from build123d import *

# Parameters (mm, degrees)
SKETCH1_W           = 40
SKETCH1_H           = 40
BOSS_EXTRUDE1_DEPTH = 10
SKETCH2_R           = 1
CUT_EXTRUDE1_DEPTH  = 11
SKETCH3_R           = 19
CUT_EXTRUDE2_DEPTH  = 11


with BuildPart() as part:
    # Sketch1 → Boss-Extrude1 (new body)
    with BuildSketch(Plane.XY):
        with Locations((20, 20)):
            Rectangle(SKETCH1_W, SKETCH1_H)
    extrude(amount=BOSS_EXTRUDE1_DEPTH)

    # Sketch2 → Cut-Extrude1 (cut, through all)
    with BuildSketch(Plane.XY.offset(10)):
        with Locations((36, 36)):
            Circle(SKETCH2_R)
        with Locations((4, 36)):
            Circle(SKETCH2_R)
        with Locations((4, 4)):
            Circle(SKETCH2_R)
        with Locations((36, 4)):
            Circle(SKETCH2_R)
    extrude(amount=-CUT_EXTRUDE1_DEPTH, mode=Mode.SUBTRACT)

    # Sketch3 → Cut-Extrude2 (cut, through all)
    with BuildSketch(Plane.XY.offset(10)):
        with Locations((20, 20)):
            Circle(SKETCH3_R)
    extrude(amount=-CUT_EXTRUDE2_DEPTH, mode=Mode.SUBTRACT)


solid = part.part
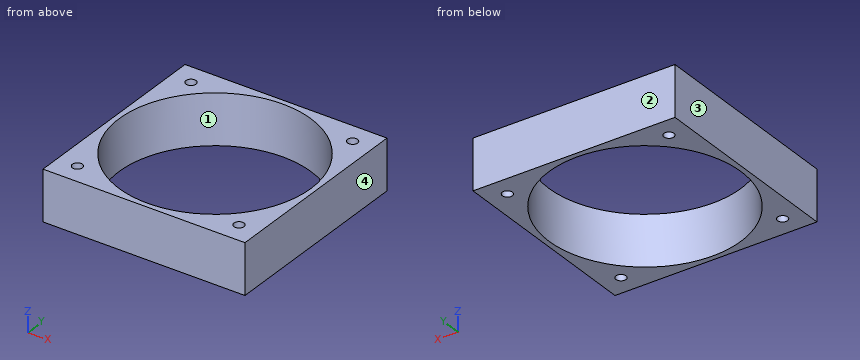
Geometry check sheet. Reference: the model listing, model coordinates, mm. Face numbers are marked on the shaded views. Round coordinates to 2 decimals unless told otherwise and drop trailing zeros. Write each loop counter-clockwise with the first axis right and the second up, starting at its lowest first coordinate (ties: lowest second). Pieces come first, ordered by that corner, then holes.
Item 1: Mould release check, pull along X, two halves, no side actions. Record for the marked faces 1, 2, 3 and 4: +X half, -X half, draft (parallel to the pull), parting line (faces both ways), or undercut.
Determined:
face 1: undercut
face 2: draft
face 3: -X half
face 4: +X half
Item 2: Section check C-C (x = 13). Record the boundary of the cut face in (y, z).
Determined:
outline: (0, 0) - (2.34, 0) - (2.34, 10) - (0, 10) - close; (37.66, 0) - (40, 0) - (40, 10) - (37.66, 10) - close
Item 3: Material ranges on line 1 along Y through (x, z) = (20, 2); line 2 along Y through (x, z) = (36, 3.25); line 3 along X through (y, z) = (5.5, 0.5), recorded low to high.
Determined:
line 1: y = 0 to 1, 39 to 40
line 2: y = 0 to 3, 5 to 9.75, 30.25 to 35, 37 to 40
line 3: x = 0 to 7.72, 32.28 to 40
Item 4: Section check A-A (z = 8.25). Record the boundary of the cut face in (x, y).
Determined:
outline: (0, 0) - (40, 0) - (40, 40) - (0, 40) - close; hole circle Ø38 at (20, 20); hole circle Ø2 at (4, 4); hole circle Ø2 at (4, 36); hole circle Ø2 at (36, 4); hole circle Ø2 at (36, 36)
Item 5: Section check D-D (x = 4). Record the boundary of the cut face in (y, z).
Determined:
outline: (0, 0) - (3, 0) - (3, 10) - (0, 10) - close; (5, 0) - (9.75, 0) - (9.75, 10) - (5, 10) - close; (30.25, 0) - (35, 0) - (35, 10) - (30.25, 10) - close; (37, 0) - (40, 0) - (40, 10) - (37, 10) - close
Item 6: Section check B-B (y = 20). Record the boundary of the cut face in (x, z).
Determined:
outline: (0, 0) - (1, 0) - (1, 10) - (0, 10) - close; (39, 0) - (40, 0) - (40, 10) - (39, 10) - close
